```python
from build123d import *

# Parameters (mm, degrees)
F1_DEPTH = 195
F2_R     = 5.682985
F3_DEPTH = 5
F4_R     = 5.682985
F5_DEPTH = 5


with BuildPart() as f1:
    # F0 (on Top) → F1 (new body)
    with BuildSketch(Plane.XY):
        Polygon((75.046803, 83.914765), (-74.953197, 83.914765), (-74.953197, 65.914765), (-68.953197, 65.914765), (-68.953197, 77.914765), (69.046803, 77.914765), (69.046803, -60.085235), (57.046803, -60.085235), (57.046803, -66.085235), (75.046803, -66.085235), align=None)
    extrude(amount=F1_DEPTH)

    # F2 (on face) → F3 (join)
    with BuildSketch(Plane.YZ.offset(75.046803)):
        with Locations((-41.085235, 170)):
            Circle(F2_R)
        with Locations((-41.085235, 100)):
            Circle(F2_R)
        with Locations((-41.085235, 30)):
            Circle(F2_R)
    extrude(amount=F3_DEPTH)

    # F4 (on face) → F5 (join)
    with BuildSketch(Plane(origin=(0, 83.914765, 0), x_dir=(-1, 0, 0), z_dir=(0, 1, 0))):
        with Locations((54.953197, 175)):
            Circle(F4_R)
        with Locations((54.953197, 105)):
            Circle(F4_R)
        with Locations((54.953197, 35)):
            Circle(F4_R)
    extrude(amount=F5_DEPTH)


solid = f1.part
```
Part model, mm, in its own coordinate system. A direction names the side the tool comes from. Give positions to 0.01 mm unless a question says otherwise; leave off trailing zeros. Loops run counter-clockwise (first coordinate to the right, second up) from the corner with the lowest first, then second, coordinate; pieces in that order, holes last. Notation, with made-up numbers: M 4,-27.75 L 53,-27.75 A23 ccw 53,-18.75 Z; hole C -30,35 d7. An arc over 180 degrees is marked long. Return JSON: item names as keys, results as strings.
1) Saw through at A-A, the plane z = 121. List the corners of the cut face in (x, y), then the cut area to 3 significant figures.
Calculated:
{"outline": "M -74.95,65.91 L -68.95,65.91 L -68.95,77.91 L 69.05,77.91 L 69.05,-60.09 L 57.05,-60.09 L 57.05,-66.09 L 75.05,-66.09 L 75.05,83.91 L -74.95,83.91 Z", "area": "1,910 mm2"}
2) Drill centre lines: line 1 (X direction, y = 77, z = 104); line 2 (Y direction, x = 63.5, z = 101); line 3 (Y direction, x = -30.5, z = 117). Where is each one in solid material? Low to high.
Calculated:
{"line 1": "x = -74.95 to -68.95, 69.05 to 75.05", "line 2": "y = -66.09 to -60.09, 77.91 to 83.91", "line 3": "y = 77.91 to 83.91"}
3) Saw through at C-C, the plane x = -6. List the corners of the cut face in (y, z).
Calculated:
{"outline": "M 77.91,0 L 83.91,0 L 83.91,195 L 77.91,195 Z"}
4) Pull direction X, two halves, no side cores. Call faces 3 (the face through (-68.953, 72, 96)), 4 (the face through (57.047, -63, 96)), 5 (the face through (80.047, -41, 100)): released by +X, released by -X, zero draft, split by the parting line, or undercut.
Calculated:
{"face 3": "undercut", "face 4": "released by -X", "face 5": "released by +X"}
5) 3-axis set-ups, long thin cutter, end or side, ignore diameter. For faces 1 (the face through (77.512, -45.595, 96.542)), 2 (the face through (-55, 88.915, 175)): which of +Z, -Z, +X, -X, +Y, -Y reach the whole face in a straight line?
Calculated:
{"face 1": "+X", "face 2": "+Z, -Z, +X, -X, +Y"}
6) Saw through at B-B, the plane y = -42. List the corners of the cut face in (x, z).
Calculated:
{"outline": "M 69.05,0 L 75.05,0 L 75.05,24.39 L 80.05,24.39 L 80.05,35.61 L 75.05,35.61 L 75.05,94.39 L 80.05,94.39 L 80.05,105.61 L 75.05,105.61 L 75.05,164.39 L 80.05,164.39 L 80.05,175.61 L 75.05,175.61 L 75.05,195 L 69.05,195 Z"}
7) Saw through at D-D, the plane y = 61. List the corners of the cut face in (x, z), then the cut area to 3 significant figures.
Calculated:
{"outline": "M 69.05,0 L 75.05,0 L 75.05,195 L 69.05,195 Z", "area": "1,170 mm2"}
8) Flat gauge pins, fed straight in: pin 1 Ø4 at (x, z) = (24.5, 66) entering from -Y; pin 2 Ø5 at (y, z) = (-63.5, 79.5) entering from -X; pin 3 Ø1 at (y, z) = (8, 158.5) entering from +X. Where does each tip first touch, or does it go through?
Calculated:
{"pin 1": "stops at y = 77.91", "pin 2": "stops at x = 57.05", "pin 3": "stops at x = 75.05"}
